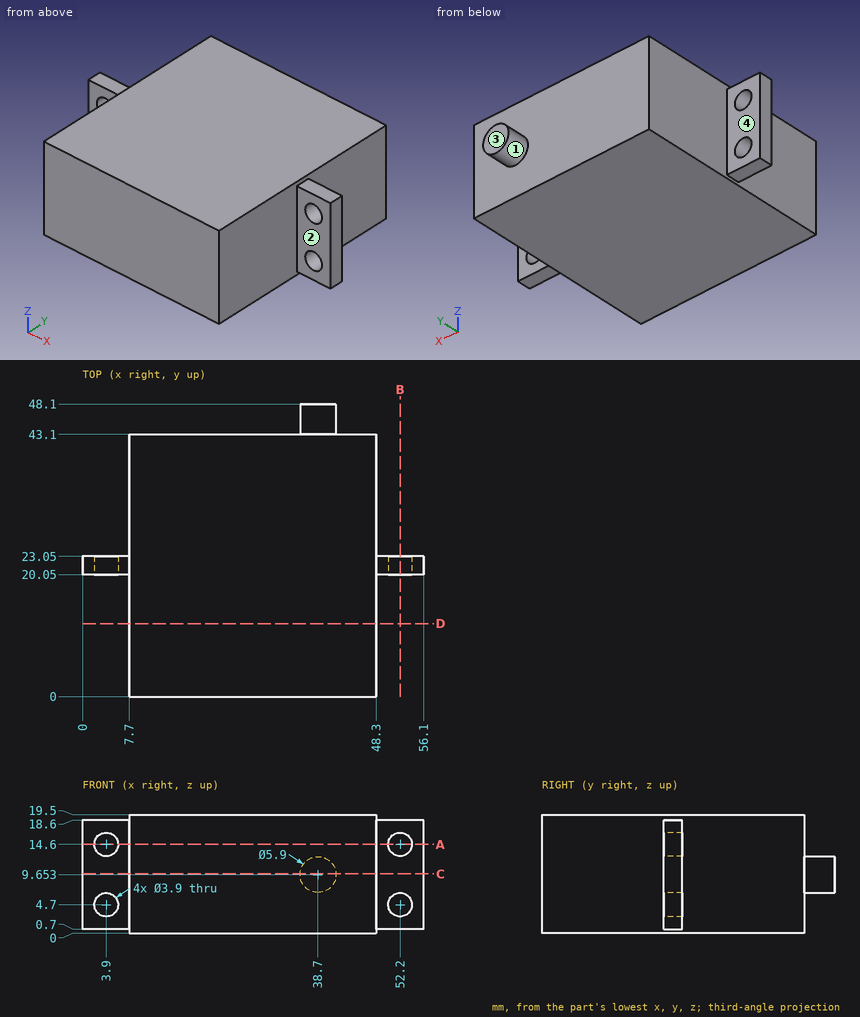
Input: dimensioned drawing with shaded views. Units: mm. Origin: part minimum x, y, z. A direction names the side the tool comes from. Give positions to 0.01 mm unless a question says otherwise; leave off trailing zeros. Order: outer loops, then holes, each group sorted by start corner. A loop starts at its lowest first (then second) coordinate and runs counter-clockwise, first axis right, second up. Notation, with made-up numbers: (-18, -22) -> (41, -22) arc R26 cw to (41, 0) -> close; hole circle Ø7 at (-13.75, 74). An arc over 180 degrees is marked (long way). Answer as a JSON object with one key per item and string values.
Q1. Material intervals for probe 1 along X at (y, z) = (21.8, 14.6); probe 2 along Z at (x, y) = (52.2, 22); probe 3 along Y at (x, z) = (42.5, 18.25), sorted ascending.
Entries:
{"probe 1": "x = 0 to 1.95, 5.85 to 50.25, 54.15 to 56.1", "probe 2": "z = 0.7 to 2.75, 6.65 to 12.65, 16.55 to 18.6", "probe 3": "y = 0 to 43.1"}
Q2. Section B-B (x = 52.2). Output: boundary loops of the cut face in (y, z), plus the area to 3 significant figures.
Entries:
{"outline": "(20.05, 0.7) -> (23.05, 0.7) -> (23.05, 2.75) -> (20.05, 2.75) -> close; (20.05, 6.65) -> (23.05, 6.65) -> (23.05, 12.65) -> (20.05, 12.65) -> close; (20.05, 16.55) -> (23.05, 16.55) -> (23.05, 18.6) -> (20.05, 18.6) -> close", "area": "30.3 mm^2"}
Q3. Section D-D (y = 12). Output: boundary loops of the cut face in (x, z).
Entries:
{"outline": "(7.7, 0) -> (48.3, 0) -> (48.3, 19.5) -> (7.7, 19.5) -> close"}
Q4. Access query for the marked faces 1, 2, 3 and 4. Directions: +Z, -Z, +X, -X, +Y, -Y. A direction counts if a zero-diameter tool reaches every point of the face in a straight line with its end or side. Return the directions, or none.
Entries:
{"face 1": "+Y", "face 2": "+Z, -Z, +X, -Y", "face 3": "+Z, -Z, +X, -X, +Y", "face 4": "+Z, -Z, -X, +Y"}
Q5. Section C-C (z = 9.75). Output: boundary loops of the cut face in (x, y).
Entries:
{"outline": "(0, 20.05) -> (7.7, 20.05) -> (7.7, 0) -> (48.3, 0) -> (48.3, 20.05) -> (56.1, 20.05) -> (56.1, 23.05) -> (48.3, 23.05) -> (48.3, 43.1) -> (41.65, 43.1) -> (41.65, 48.1) -> (35.75, 48.1) -> (35.75, 43.1) -> (7.7, 43.1) -> (7.7, 23.05) -> (0, 23.05) -> close"}
Q6. First-contact query: pin 1 (1.5 mm diameter, centred on x = 53.5, y = 21.5, fed in from +Z); pin 2 (1.5 mm diameter, centred on x = 32.5, z = 5, fed in from -Y); pin 3 (6 mm diameter, centred on x = 3.9, z = 14.6, fed in from +Y); pin 4 (4 mm diameter, centred on y = 17, z = 3.5, fed in from +X). Flat tips, straight axial feed; report the tip coordinate or a pass-through.
Entries:
{"pin 1": "stops at z = 18.6", "pin 2": "stops at y = 0", "pin 3": "stops at y = 23.05", "pin 4": "stops at x = 48.3"}
Q7. Section A-A (z = 14.6). Output: boundary loops of the cut face in (x, y).
Entries:
{"outline": "(0, 20.05) -> (1.95, 20.05) -> (1.95, 23.05) -> (0, 23.05) -> close; (5.85, 20.05) -> (7.7, 20.05) -> (7.7, 0) -> (48.3, 0) -> (48.3, 20.05) -> (50.25, 20.05) -> (50.25, 23.05) -> (48.3, 23.05) -> (48.3, 43.1) -> (7.7, 43.1) -> (7.7, 23.05) -> (5.85, 23.05) -> close; (54.15, 20.05) -> (56.1, 20.05) -> (56.1, 23.05) -> (54.15, 23.05) -> close"}
